The figure shows three views and two pictorial views of one solid part (mm, origin at its lowest corner). Answer the questions. Coordinates: 2 decimals unless noted, no trailing zeros. Order: outer loops, then holes, each group sorted by start corner. A loop starts at its lowest first (then second) coordinate and runs counter-clockwise, first axis right, second up.
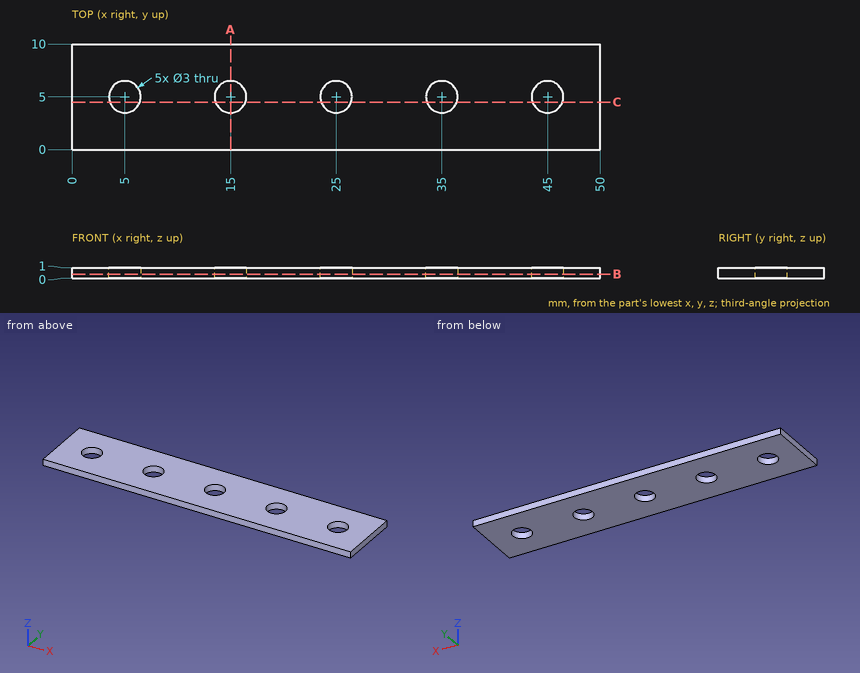
Q1. The part is cut by section C-C, the plane y = 4.5. Determine the outline of the cut face in (x, z).
Q2. The part is cut by section B-B, the plane z = 0.4. Determine the outline of the cut face in (x, y).
Q3. The part is cut by section A-A, the plane x = 15. Determine the outline of the cut face in (y, z), then the cut area to 3 significant figures.
Q4. Straight lines are drawn through the part: L1, parallel to Y at x = 35, z = 0.45; L2, parallel to X at y = 6, z = 0.15; L3, parallel to X at y = 5.5, z = 0.1. For each, find the intervals that lie inside material, in ascending order.
Computed values:
1. outline: (0, 0) - (3.59, 0) - (3.59, 1) - (0, 1) - close; (6.41, 0) - (13.59, 0) - (13.59, 1) - (6.41, 1) - close; (16.41, 0) - (23.59, 0) - (23.59, 1) - (16.41, 1) - close; (26.41, 0) - (33.59, 0) - (33.59, 1) - (26.41, 1) - close; (36.41, 0) - (43.59, 0) - (43.59, 1) - (36.41, 1) - close; (46.41, 0) - (50, 0) - (50, 1) - (46.41, 1) - close
2. outline: (0, 0) - (50, 0) - (50, 10) - (0, 10) - close; hole circle Ø3 at (5, 5); hole circle Ø3 at (15, 5); hole circle Ø3 at (25, 5); hole circle Ø3 at (35, 5); hole circle Ø3 at (45, 5)
3. outline: (0, 0) - (3.5, 0) - (3.5, 1) - (0, 1) - close; (6.5, 0) - (10, 0) - (10, 1) - (6.5, 1) - close
3. area: 7.00 mm2
4. L1: y = 0 to 3.5, 6.5 to 10
4. L2: x = 0 to 3.88, 6.12 to 13.88, 16.12 to 23.88, 26.12 to 33.88, 36.12 to 43.88, 46.12 to 50
4. L3: x = 0 to 3.59, 6.41 to 13.59, 16.41 to 23.59, 26.41 to 33.59, 36.41 to 43.59, 46.41 to 50
